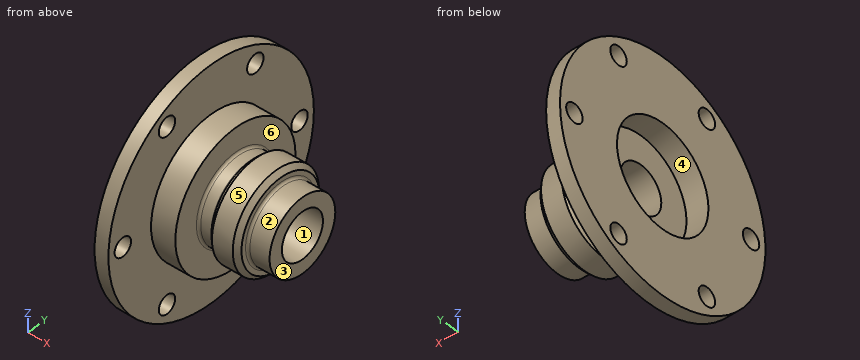
from build123d import *

# Parameters (mm, degrees)
SKETCH2_W     = 9.5
SKETCH2_H     = 22.25
SKETCH2_W_2   = 36
SKETCH2_H_2   = 10
HOLE1_D       = 8
CHAMFER1_SIZE = 2
FILLET1_R     = 1


with BuildPart() as part:
    # Sketch1 → Revolve1 (revolve)
    with BuildSketch(Plane.XY):
        Polygon((0, 0), (0, 50), (6, 50), (6, 29.25), (16.5, 29.25), (16.5, 18), (23, 18), (23, 21), (36, 21), (36, 16), (45.5, 16), (45.5, 0), align=None)
    revolve(axis=Axis((45.5, 0, 0), (-1, 0, 0)))

    # Sketch2 → Cut-Revolve1 (revolve, cut)
    with BuildSketch(Plane.XY, mode=Mode.PRIVATE) as cut_revolve1_sk:
        with Locations((4.75, 11.125)):
            Rectangle(SKETCH2_W, SKETCH2_H)
        with Locations((27.5, 5)):
            Rectangle(SKETCH2_W_2, SKETCH2_H_2)
    revolve(cut_revolve1_sk.sketch.rotate(Axis((0, 0, 0), (1, 0, 0)), 90), axis=Axis((0, 0, 0), (1, 0, 0)), mode=Mode.SUBTRACT)

    # Hole1 (through all)
    with Locations(Plane.ZY):
        with Locations((0, 0), (0, 43), (37.239092363, 21.5), (37.239092363, -21.5), (0, -43), (-37.239092363, -21.5), (-37.239092363, 21.5)):
            Hole(HOLE1_D / 2)

    # Chamfer1
    chamfer1_edges = [part.edges().sort_by_distance(p)[0] for p in [
        (36, -21, 0),
        (23, -21, 0),
    ]]
    chamfer(chamfer1_edges, length=CHAMFER1_SIZE)

    # Fillet1
    fillet1_edges = [part.edges().sort_by_distance(p)[0] for p in [
        (36, -16, 0),
        (23, -18, 0),
        (16.5, -18, 0),
    ]]
    fillet(fillet1_edges, radius=FILLET1_R - 0.0001)  # a hair under: the kernel refuses the full size


solid = part.part
CAD build for the part. Positions are in the model's coordinates, mm. Face numbers are marked on the shaded views. A direction names the side the tool comes from. Round coordinates to 2 decimals unless told otherwise and drop trailing zeros. Write each loop counter-clockwise with the first axis right and the second up, starting at its lowest first coordinate (ties: lowest second). Pieces come first, ordered by that corner, then holes. Notation, with made-up numbers: M -36.75,32.25 L -6.75,32.25 A11 ccw -6.75,53.25 Z; hole C -7,-26.5 d2. An arc over 180 degrees is marked long. Put each result on its own line as item: value. Start each with the question number.
1) Saw through at C-C, the plane y = -43. Write the cut outline in (x, z).
2) Saw through at B-B, the plane x = 41. Write the cut outline in (y, z), and give its area (3 significant figures).
3) Saw through at A-A, the plane z = -37. Write the cut outline in (x, y).
4) Pull direction Z, two halves, no side cores. Call the marked faces 1, 2 and 3: pulls with the +Z half, pulls with the -Z half, needs draft (parallel to the pull), parting line crosses it, or undercut.
5) Saw through at D-D, the plane y = -28. Write the cut outline in (x, z).
6) Drill centre lines: probe 1 along Y at (x, z) = (2, 0); probe 2 along Y at (x, z) = (29.5, 0); probe 3 along X at (y, z) = (-33, -4). Where is each one in solid material? Low to high. Write a range as [from, to].
7) Pin check, flat tips, straight feed: pin 1 Ø5 at (x, y) = (40.5, -4.5) entering from -Z; pin 2 Ø13.5 at (y, z) = (1, -5.5) entering from -X; pin 3 Ø5 at (x, z) = (7.5, -16) entering from -Y. Stop position of each tip, or through.
8) 3-axis set-ups, long thin cutter, end or side, ignore diameter. For the marked faces 4, 5 and 6: which of +Z, -Z, +X, -X, +Y, -Y reach the whole face in a straight line?
Resolved:
1. outline: M 0,-25.51 L 6,-25.51 L 6,-4 L 0,-4 Z; M 0,4 L 6,4 L 6,25.51 L 0,25.51 Z
2. outline: C 0,0 d32; hole C 0,0 d20
2. area: 490 mm²
3. outline: M 0,-33.63 L 6,-33.63 L 6,-25.49 L 0,-25.49 Z; M 0,-17.51 L 6,-17.51 L 6,17.51 L 0,17.51 Z; M 0,25.49 L 6,25.49 L 6,33.63 L 0,33.63 Z
4. face 1: undercut
4. face 2: parting line crosses it
4. face 3: needs draft
5. outline: M 0,-41.42 L 6,-41.42 L 6,-8.46 L 16.5,-8.46 L 16.5,8.46 L 6,8.46 L 6,41.42 L 0,41.42 Z
6. probe 1: [-50, -47], [-39, -22.25], [22.25, 39], [47, 50]
6. probe 2: [-21, -10], [10, 21]
6. probe 3: [0, 6]
7. pin 1: z = -15.87
7. pin 2: x = 9.5
7. pin 3: y = -48
8. face 4: -X
8. face 5: +X
8. face 6: none
